Geometry: final body of the model. Coordinates: model frame, mm. A direction names the side the tool comes from. Coordinates: 2 decimals unless noted, no trailing zeros. Order: outer loops, then holes, each group sorted by start corner. A loop starts at its lowest first (then second) coordinate and runs counter-clockwise, first axis right, second up. Notation, with made-up numbers: M 7,36.5 L 20,36.5 A24 ccw 20,60.5 Z; hole C 19,-2.75 d10. An arc over 180 degrees is marked long. Use CSV: the item, a comma, the result in double quotes. Start each with the question number.
Q1. Section query B-B, the plane x = -1.75. Output: boundary loops of the cut face in (y, z).
Q2. Section query C-C, the plane z = -11. Output: boundary loops of the cut face in (x, y), and give its area (3 significant figures).
Q3. Section query D-D, the plane z = 9.25. Output: boundary loops of the cut face in (x, y).
Q4. Access query for faces 4 (the face through (-8.15, 9, -8)), 5 (the face through (-14.056, 2.681, 6.466)), 6 (the face through (-18, 0, 0)). Directions: +Z, -Z, +X, -X, +Y, -Y. A direction counts if a zero-diameter tool reaches every point of the face in a straight line with its end or side. Return the directions, or none.
Q5. Section query A-A, the plane y = -6. Output: boundary loops of the cut face in (x, z), and give its area (3 significant figures).
Q6. First-contact query: P1, Ø1.5, axis at x = -8.5, z = -1.5, coming from the -Y side; P2, Ø3, axis at x = -2.5, y = -0.5, coming from the -Z side; P3, Ø4, axis at x = -12.5, z = -3.5, coming from the +Y side; P4, Ø4, axis at y = 8.5, z = -2.5, coming from the -X side. Flat tips, straight axial feed; report the tip coordinate or a pass-through.
Q7. Mould query, pull axis X, two halves, no side actions, for faces 1 (the face through (-15.49, -0.51, 0.11)), 2 (the face through (8.15, 9, 8)), 3 (the face through (-2, 0, -3)). Classes: +X half, -X half, draft (parallel to the pull), parting line (faces both ways), or undercut.
Q8. Ray query, probe 1 along Y at (x, z) = (-4.25, 0); probe 2 along Y at (x, z) = (-8.75, 0). Return the intervals inside material, ascending.
from build123d import *

# Parameters (mm, degrees)
F_6_0_6_DIAMETER_HOLE2_D     = 6
F_6_0_6_DIAMETER_HOLE2_DEPTH = 24
F_6_0_6_DIAMETER_HOLE2_TIP   = 1.802581857


with BuildPart() as part:
    # Sketch1 → Revolve1 (revolve)
    with BuildSketch(Plane(origin=(0, 0, 0), x_dir=(1, 0, 0), z_dir=(0, 1, 0))):
        Polygon((0, -11.46), (-8.15, -11.46), (-8.15, -13), (-10, -13), (-10, -7), (-18, -7), (-18, 0), (-10, 0), (10, 0), (10, -13), (8.15, -13), (8.15, -11.46), align=None)
    revolve(axis=Axis((-10, 0, 0), (1, 0, 0)))

    # Ø6.0 (6) Diameter Hole2
    with Locations(Plane(origin=(10, 0, 0), x_dir=(0, 0, -1), z_dir=(1, 0, 0))):
        with Locations((0, 0)):
            Hole(F_6_0_6_DIAMETER_HOLE2_D / 2, depth=F_6_0_6_DIAMETER_HOLE2_DEPTH)
            with Locations((0, 0, -(F_6_0_6_DIAMETER_HOLE2_DEPTH + F_6_0_6_DIAMETER_HOLE2_TIP / 2))):  # 118° drill point
                Cone(0, F_6_0_6_DIAMETER_HOLE2_D / 2, F_6_0_6_DIAMETER_HOLE2_TIP, mode=Mode.SUBTRACT)


solid = part.part
Responses:
1,outline,"C 0,0 d22.92; hole C 0,0 d6"
2,outline,"M -10,-6.93 L -8.15,-6.93 L -8.15,-3.21 L 8.15,-3.21 L 8.15,-6.93 L 10,-6.93 L 10,6.93 L 8.15,6.93 L 8.15,3.21 L -8.15,3.21 L -8.15,6.93 L -10,6.93 Z"
2,area,"156 mm²"
3,outline,"M -10,-9.13 L -8.15,-9.13 L -8.15,-6.77 L 8.15,-6.77 L 8.15,-9.13 L 10,-9.13 L 10,9.13 L 8.15,9.13 L 8.15,6.77 L -8.15,6.77 L -8.15,9.13 L -10,9.13 Z"
4,face 4,"none"
4,face 5,"-X"
4,face 6,"+Z, -Z, -X, +Y, -Y"
5,outline,"M -18,-3.61 L -10,-3.61 L -10,-11.53 L -8.15,-11.53 L -8.15,-9.76 L 8.15,-9.76 L 8.15,-11.53 L 10,-11.53 L 10,11.53 L 8.15,11.53 L 8.15,9.76 L -8.15,9.76 L -8.15,11.53 L -10,11.53 L -10,3.61 L -18,3.61 Z"
5,area,"461 mm²"
6,P1,"stops at y = -12.98"
6,P2,"stops at z = -11.46"
6,P3,"stops at y = 6.84"
6,P4,"stops at x = -18"
7,face 1,"+X half"
7,face 2,"undercut"
7,face 3,"draft"
8,probe 1,"y = -11.46 to -3, 3 to 11.46"
8,probe 2,"y = -13 to -3, 3 to 13"
